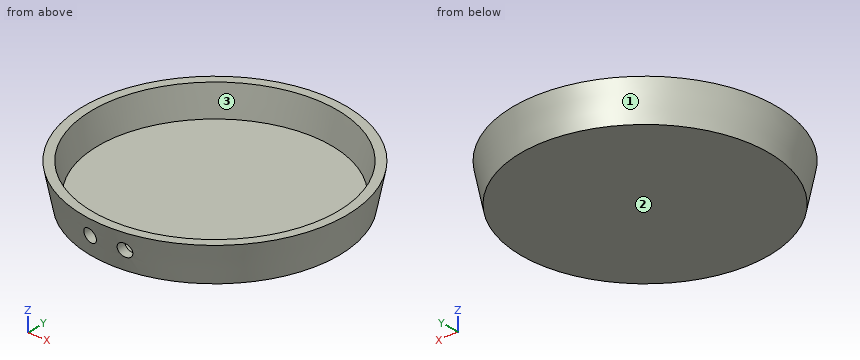
```python
from build123d import *

# Parameters (mm, degrees)
F3_R     = 3
F4_DEPTH = 15


with BuildPart() as f1:
    # F0 (on Front) → F1 (revolve)
    with BuildSketch(Plane.XZ):
        Polygon((50, 0), (0, 0), (0, -3.81), (53.123453, -3.81), (56.385453, 12.5), (52.5, 12.5), align=None)
    revolve(axis=Axis((0, 0, 6.25), (0, 0, 1)))

    # F3 (on offset) → F4 (cut)
    with BuildSketch(Plane.XZ.offset(56.5)):
        with Locations((7.5, 5)):
            Circle(F3_R)
        with Locations((-7.5, 5)):
            Circle(F3_R)
    extrude(amount=-F4_DEPTH, mode=Mode.SUBTRACT)


solid = f1.part
```
Part model, mm, in its own coordinate system. Face numbers are marked on the shaded views. Give positions to 0.01 mm unless a question says otherwise; leave off trailing zeros. Write each loop counter-clockwise with the first axis right and the second up, starting at its lowest first coordinate (ties: lowest second). Pieces come first, ordered by that corner, then holes. Notation, with made-up numbers: (62.25, -37.75) -> (103.25, -37.75) arc R29 ccw to (103.25, -0.75) -> close; hole circle Ø1 at (-34, 27). An arc over 180 degrees is marked (long way). Put each result on its own line as item: value. Start each with the question number.
Item 1: Pull direction Y, two halves, no side cores. Call the marked faces 1, 2 and 3: pulls with the +Y half, pulls with the -Y half, needs draft (parallel to the pull), parting line crosses it, or undercut.
Item 2: Cut at A-A (z = 5). List the corners of the cut face in (x, y), then the cut area to 3 significant figures.
Item 3: Cut at B-B (y = 0). List the corners of the cut face in (x, z), then the cut area to 3 significant figures.
Item 4: Pin check, flat tips, straight feed: pin 1 Ø2 at (x, z) = (-23, 1.5) entering from -Y; pin 2 Ø1 at (x, z) = (0.5, 11) entering from +Y; pin 3 Ø3.5 at (x, z) = (7.5, 5) entering from -Y. Stop position of each tip, or through.
Item 5: Wall check: L1, parallel to Z at x = 7.5, y = -52.5; L2, parallel to Z at x = -22.5, y = 27; L3, parallel to Y at x = 26.5, z = 3. Give the ranges that are in metal, low to high. Write a range as [from, to].
Answer list:
1. face 1: parting line crosses it
1. face 2: needs draft
1. face 3: undercut
2. outline: (-10.5, -53.87) -> (-10.5, -49.91) arc R51 cw (long way) to (10.5, -49.91) -> (10.5, -53.87) arc R54.89 ccw (long way) to start; (-4.5, -54.7) arc R54.89 ccw to (4.5, -54.7) -> (4.5, -50.8) arc R51 cw to (-4.5, -50.8) -> close
2. area: 1,250 mm2
3. outline: (-56.39, 12.5) -> (-53.12, -3.81) -> (53.12, -3.81) -> (56.39, 12.5) -> (52.5, 12.5) -> (50, 0) -> (-50, 0) -> (-52.5, 12.5) -> close
3. area: 505 mm2
4. pin 1: stops at y = -49.57
4. pin 2: stops at y = 56.18
4. pin 3: stops at y = 49.99
5. L1: z = [-3.81, 2], [8, 12.5]
5. L2: z = [-3.81, 0]
5. L3: y = [-47.61, -43.11], [43.11, 47.61]
